Verification items for the finished model (mm, model axes). A direction names the side the tool comes from. Give positions to 0.01 mm unless a question says otherwise; leave off trailing zeros. Loops run counter-clockwise (first coordinate to the right, second up) from the corner with the lowest first, then second, coordinate; pieces in that order, holes last. Notation, with made-up numbers: (47.5, 32.25) - (72.5, 32.25) arc R16 ccw to (72.5, 58.25) - close; hole circle Ø10 at (46.25, 41). An arc over 180 degrees is marked (long way). One line per question, with ' | ' between items. Start each with the question number.
1. Section check C-C, the plane y = 60.96. Enter the section's corners in (x, z), then the cut area to 3 significant figures.
2. Mould release check, pull along Z, two halves, no side actions. Record for faces 1 (the face through (0, 63, 13.97)), 2 (the face through (12.718, 19.766, -2.93)), 3 (the face through (12.718, 49.476, 0.827)), 4 (the face through (13.97, 62.6, 6.4)): +Z half, -Z half, draft (parallel to the pull), parting line (faces both ways), or undercut.
3. Tool access check on faces 5 (the face through (-13.97, 63, 0)), 6 (the face through (0, 64, -11.43)), 7 (the face through (12.72, 72.54, 1.38)), 8 (the face through (12, 0, 0)), 9 (the face through (28.194, 132, 153)). Record the directions out of +Z, -Z, +X, -X, +Y, -Y that give a thin tool (end or side, any length) a straight path to the whole face; none if there is none.
4. Section check A-A, the plane z = 0. State how many separate pieces and enclosed holes the cut face has, then the cut area to 3 significant figures.
5. Section check D-D, the plane x = -104. Enter the section's corners in (y, z).
6. Depth check by flat-ended pin: pin 1 Ø11.5 at (x, z) = (-3.5, -1.5) entering from -Y; pin 2 Ø16.5 at (y, z) = (60.96, 0) entering from +X; pin 3 Ø20.5 at (y, z) = (43.18, 0) entering from -X. Enter the tip coordinate at first touch or a pass-through.
7. Section check B-B, the plane y = 119. Enter the section's corners in (x, z).
8. Thickness scan on line 1 along Y through (x, z) = (12.25, 0); line 2 along Z through (x, y) = (12, 25); line 3 along Y through (x, z) = (-334.5, 23). Record the ranges inside material, lowest first. Write a range as from..to.
from build123d import *

# Parameters (mm, degrees)
SKETCH1_W           = 27.94
SKETCH1_H           = 27.94
BOSS_EXTRUDE1_DEPTH = 127
CUT_EXTRUDE1_REACH  = 130.528
SKETCH2_W           = 22.86
SKETCH2_H           = 22.86
SKETCH3_W           = 381
SKETCH3_H           = 330.2
BOSS_EXTRUDE2_DEPTH = 10.16
CUT_EXTRUDE2_REACH  = 515.785
SKETCH4_R           = 6.35
SKETCH5_W           = 330.2
SKETCH5_H           = 10.16
BOSS_EXTRUDE3_DEPTH = 203.2
SKETCH7_R           = 7.5
CUT_EXTRUDE4_DEPTH  = 5.08
SKETCH8_W           = 330.2
SKETCH8_H           = 10.16
CUT_EXTRUDE5_DEPTH  = 188.976


with BuildPart() as part:
    # Sketch1 → Boss-Extrude1 (new body)
    with BuildSketch(Plane(origin=(0, 0, 0), x_dir=(1, 0, 0), z_dir=(0, 1, 0))):
        Rectangle(SKETCH1_W, SKETCH1_H)
    extrude(amount=BOSS_EXTRUDE1_DEPTH)

    # Sketch2 → Cut-Extrude1 (cut, up to next)
    with BuildSketch(Plane(origin=(0, 127, 0), x_dir=(1, 0, 0), z_dir=(0, 1, 0)), mode=Mode.PRIVATE) as cut_extrude1_sk1:
        Rectangle(SKETCH2_W, SKETCH2_H)
    cut_extrude1_tool1 = extrude(cut_extrude1_sk1.sketch, amount=-CUT_EXTRUDE1_REACH, mode=Mode.PRIVATE) & part.part
    add(cut_extrude1_tool1.solids().sort_by_distance((0, 127, 0))[0], mode=Mode.SUBTRACT)

    # Sketch3 → Boss-Extrude2 (add)
    with BuildSketch(Plane(origin=(0, 127, 0), x_dir=(1, 0, 0), z_dir=(0, 1, 0))):
        with Locations((-176.53, -151.13)):
            Rectangle(SKETCH3_W, SKETCH3_H)
    extrude(amount=BOSS_EXTRUDE2_DEPTH)

    # Sketch4 → Cut-Extrude2 (cut, up to next)
    with BuildSketch(Plane(origin=(13.97, 0, 0), x_dir=(0, 0, -1), z_dir=(1, 0, 0)), mode=Mode.PRIVATE) as cut_extrude2_sk1:
        with Locations((0, 25.4)):
            Circle(SKETCH4_R)
    cut_extrude2_tool1 = extrude(cut_extrude2_sk1.sketch, amount=-CUT_EXTRUDE2_REACH, mode=Mode.PRIVATE) & part.part
    # Sketch4 → Cut-Extrude2 (cut, up to next)
    with BuildSketch(Plane(origin=(13.97, 0, 0), x_dir=(0, 0, -1), z_dir=(1, 0, 0)), mode=Mode.PRIVATE) as cut_extrude2_sk2:
        with Locations((0, 43.18)):
            Circle(SKETCH4_R)
    cut_extrude2_tool2 = extrude(cut_extrude2_sk2.sketch, amount=-CUT_EXTRUDE2_REACH, mode=Mode.PRIVATE) & part.part
    # Sketch4 → Cut-Extrude2 (cut, up to next)
    with BuildSketch(Plane(origin=(13.97, 0, 0), x_dir=(0, 0, -1), z_dir=(1, 0, 0)), mode=Mode.PRIVATE) as cut_extrude2_sk3:
        with Locations((0, 60.96)):
            Circle(SKETCH4_R)
    cut_extrude2_tool3 = extrude(cut_extrude2_sk3.sketch, amount=-CUT_EXTRUDE2_REACH, mode=Mode.PRIVATE) & part.part
    # Sketch4 → Cut-Extrude2 (cut, up to next)
    with BuildSketch(Plane(origin=(13.97, 0, 0), x_dir=(0, 0, -1), z_dir=(1, 0, 0)), mode=Mode.PRIVATE) as cut_extrude2_sk4:
        with Locations((0, 78.74)):
            Circle(SKETCH4_R)
    cut_extrude2_tool4 = extrude(cut_extrude2_sk4.sketch, amount=-CUT_EXTRUDE2_REACH, mode=Mode.PRIVATE) & part.part
    # Sketch4 → Cut-Extrude2 (cut, up to next)
    with BuildSketch(Plane(origin=(13.97, 0, 0), x_dir=(0, 0, -1), z_dir=(1, 0, 0)), mode=Mode.PRIVATE) as cut_extrude2_sk5:
        with Locations((0, 96.52)):
            Circle(SKETCH4_R)
    cut_extrude2_tool5 = extrude(cut_extrude2_sk5.sketch, amount=-CUT_EXTRUDE2_REACH, mode=Mode.PRIVATE) & part.part
    add(cut_extrude2_tool1.solids().sort_by_distance((13.97, 25.4, 0))[0], mode=Mode.SUBTRACT)
    add(cut_extrude2_tool2.solids().sort_by_distance((13.97, 43.18, 0))[0], mode=Mode.SUBTRACT)
    add(cut_extrude2_tool3.solids().sort_by_distance((13.97, 60.96, 0))[0], mode=Mode.SUBTRACT)
    add(cut_extrude2_tool4.solids().sort_by_distance((13.97, 78.74, 0))[0], mode=Mode.SUBTRACT)
    add(cut_extrude2_tool5.solids().sort_by_distance((13.97, 96.52, 0))[0], mode=Mode.SUBTRACT)

    # Sketch5 → Boss-Extrude3 (add)
    with BuildSketch(Plane(origin=(13.97, 0, 0), x_dir=(0, 0, -1), z_dir=(1, 0, 0))):
        with Locations((-151.13, 132.08)):
            Rectangle(SKETCH5_W, SKETCH5_H)
    extrude(amount=BOSS_EXTRUDE3_DEPTH)

    # Sketch7 → Cut-Extrude4 (cut)
    with BuildSketch(Plane.XZ.offset(-127)):
        with Locations(Location((90.17, 43.501665218, 0), (0, 0, 270))):
            Circle(SKETCH7_R)
    extrude(amount=-CUT_EXTRUDE4_DEPTH, mode=Mode.SUBTRACT)

    # Sketch8 → Cut-Extrude5 (cut)
    with BuildSketch(Plane(origin=(217.17, 0, 0), x_dir=(0, 0, -1), z_dir=(1, 0, 0))):
        with Locations((-151.13, 132.08)):
            Rectangle(SKETCH8_W, SKETCH8_H)
    extrude(amount=-CUT_EXTRUDE5_DEPTH, mode=Mode.SUBTRACT)


solid = part.part
Results list:
1) outline: (-13.97, -13.97) - (13.97, -13.97) - (13.97, -6.35) - (11.43, -6.35) - (11.43, -11.43) - (-11.43, -11.43) - (-11.43, 11.43) - (11.43, 11.43) - (11.43, 6.35) - (13.97, 6.35) - (13.97, 13.97) - (-13.97, 13.97) - close | area: 226 mm²
2) face 1: +Z half | face 2: undercut | face 3: undercut | face 4: draft
3) face 5: +Z, -Z, -X, -Y | face 6: -Y | face 7: +X | face 8: +Z, -Z, +X, -X, -Y | face 9: +Z, -Z, +X, +Y, -Y
4) separate pieces: 6 | enclosed holes: 0 | area: 4,500 mm²
5) outline: (127, -13.97) - (137.16, -13.97) - (137.16, 316.23) - (127, 316.23) - close
6) pin 1: y = 127 | pin 2: x = 13.97 | pin 3: x = -13.97
7) outline: (-13.97, -13.97) - (13.97, -13.97) - (13.97, 13.97) - (-13.97, 13.97) - close; hole (-11.43, -11.43) - (11.43, -11.43) - (11.43, 11.43) - (-11.43, 11.43) - close
8) line 1: 0..19.05, 31.75..36.83, 49.53..54.61, 67.31..72.39, 85.09..90.17, 102.87..137.16 | line 2: -13.97..-6.34, 6.34..13.97 | line 3: 127..137.16
